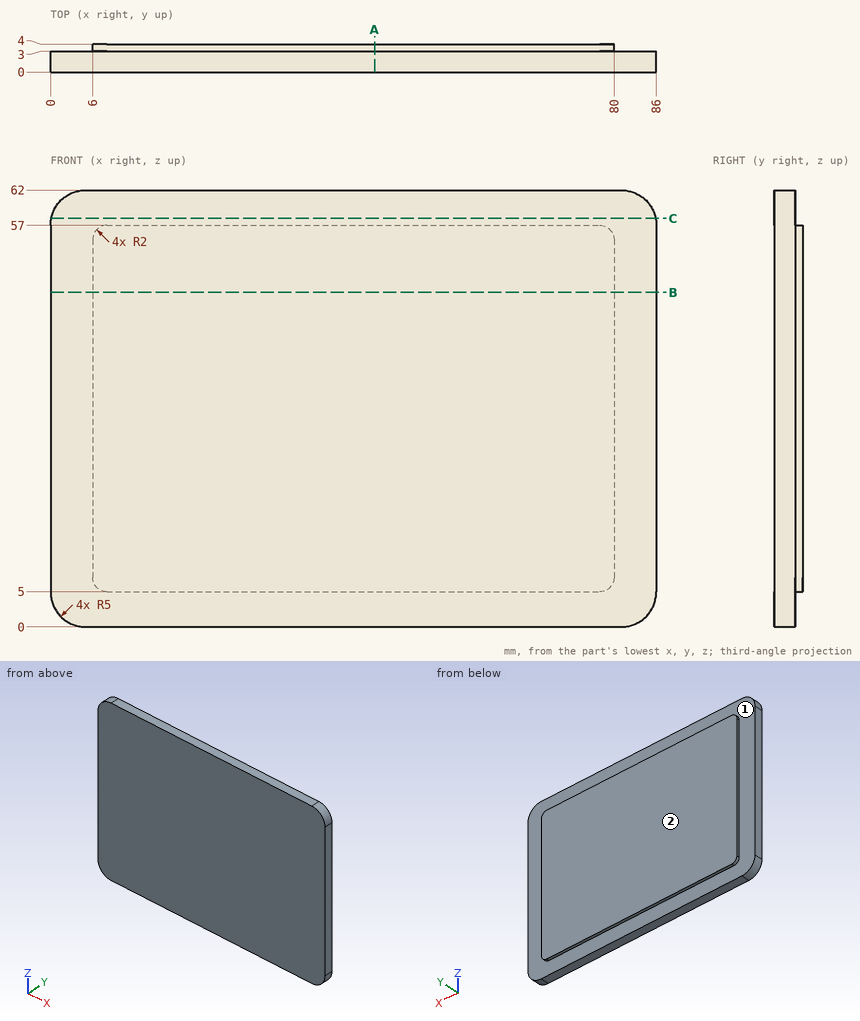
Study the drawing (mm; zero at the part's minimum x, y, z) and answer. A direction names the side the tool comes from. Coordinates: 2 decimals unless noted, no trailing zeros. Write each loop counter-clockwise with the first axis right and the second up, starting at its lowest first coordinate (ties: lowest second). Pieces come first, ordered by that corner, then holes.
Q1. A cutting plane is placed at A-A, the plane x = 46. Give the vertices of the cut face in (y, z).
Q2. A cutting plane is placed at C-C, the plane z = 58. Give the vertices of the cut face in (x, y), then the cut area to 3 significant figures.
Q3. Find the intervals of material crossed by line 1 (X direction, y = 3.6, z = 8); line 2 (Z direction, x = 45.5, y = 3.4); line 3 (Y direction, x = 82, z = 24), in increasing order.
Q4. A cutting plane is placed at B-B, the plane z = 47.5. Give the vertices of the cut face in (x, y).
Q5. Which of the six approach directions +Z, -Z, +X, -X, +Y, -Y give full straight-line access (tool end or side, diameter ignored) to the marked faces 1 and 2?
Q6. Each of these flat-tipped pins is pushed along its axis until it touches: pin 1 Ø1 at (x, y) = (23.5, 1.5) entering from -Z; pin 2 Ø0.8 at (y, z) = (3.5, 31.5) entering from +X; pin 3 Ø0.8 at (x, y) = (42, 3.5) entering from -Z. Where does it stop, or does it pass through?
Findings below:
1. outline: (0, 0) - (3, 0) - (3, 5) - (4, 5) - (4, 57) - (3, 57) - (3, 62) - (0, 62) - close
2. outline: (0.1, 0) - (85.9, 0) - (85.9, 3) - (0.1, 3) - close
2. area: 257 mm2
3. line 1: x = 6 to 80
3. line 2: z = 5 to 57
3. line 3: y = 0 to 3
4. outline: (0, 0) - (86, 0) - (86, 3) - (80, 3) - (80, 4) - (6, 4) - (6, 3) - (0, 3) - close
5. face 1: +Y
5. face 2: +Z, -Z, +X, -X, +Y
6. pin 1: stops at z = 0
6. pin 2: stops at x = 80
6. pin 3: stops at z = 5
